Part print with two shaded views. Sizes in mm from the minimum x, y, z corner. Round coordinates to 2 decimals unless told otherwise and drop trailing zeros. Order: outer loops, then holes, each group sorted by start corner. A loop starts at its lowest first (then second) coordinate and runs counter-clockwise, first axis right, second up. Notation, with made-up numbers: M 72,-26.5 L 89,-26.5 A4 ccw 89,-22.5 Z; hole C -31.5,21 d11. An arc over 180 degrees is marked long. Return JSON: item names as keys, results as strings. Group by question number.
Item 1: Slice it at A-A on x = 1.2. Write the cut outline in (y, z).
Item 2: Slice it at B-B on y = 109.5. Write the cut outline in (x, z).
Item 3: Pin check, flat tips, straight feed: pin 1 Ø10 at (y, z) = (64.5, 76) entering from -X; pin 2 Ø2.5 at (x, z) = (2.5, 50.5) entering from -Y; pin 3 Ø1.5 at (x, y) = (1.5, 100) entering from +Z. Stop position of each tip, or through.
Item 4: Probe line 1 along Z through (x, y) = (3.75, 82.5); line 2 along Y through (x, z) = (1.95, 54); line 3 along Z through (x, y) = (1.9, 106.5). List the from-to ranges inside material, lowest first.
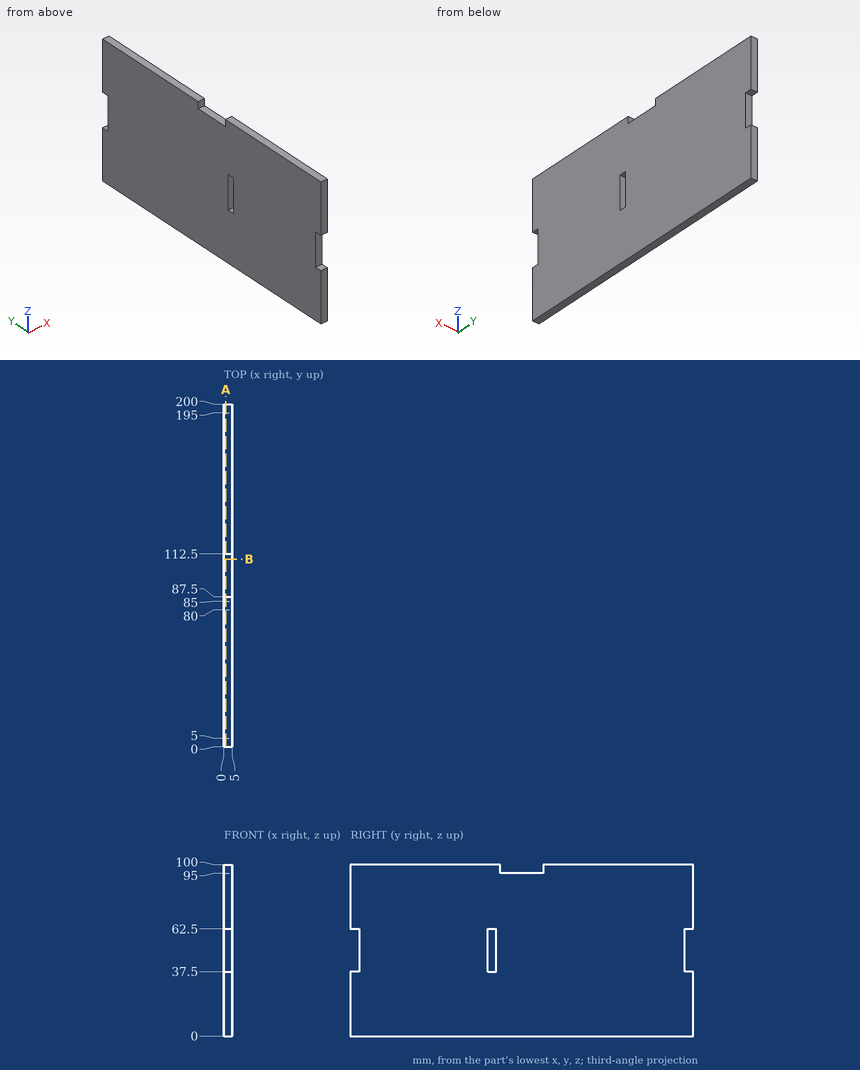
Output values:
{
 "1": {"outline": "M 0,0 L 200,0 L 200,37.5 L 195,37.5 L 195,62.5 L 200,62.5 L 200,100 L 112.5,100 L 112.5,95 L 87.5,95 L 87.5,100 L 0,100 L 0,62.5 L 5,62.5 L 5,37.5 L 0,37.5 Z; hole M 80,37.5 L 85,37.5 L 85,62.5 L 80,62.5 Z"},
 "2": {"outline": "M 0,0 L 5,0 L 5,95 L 0,95 Z"},
 "3": {"pin 1": "x = 0", "pin 2": "y = 5", "pin 3": "z = 95"},
 "4": {"line 1": "0 to 37.5, 62.5 to 100", "line 2": "5 to 80, 85 to 195", "line 3": "0 to 95"}
}
